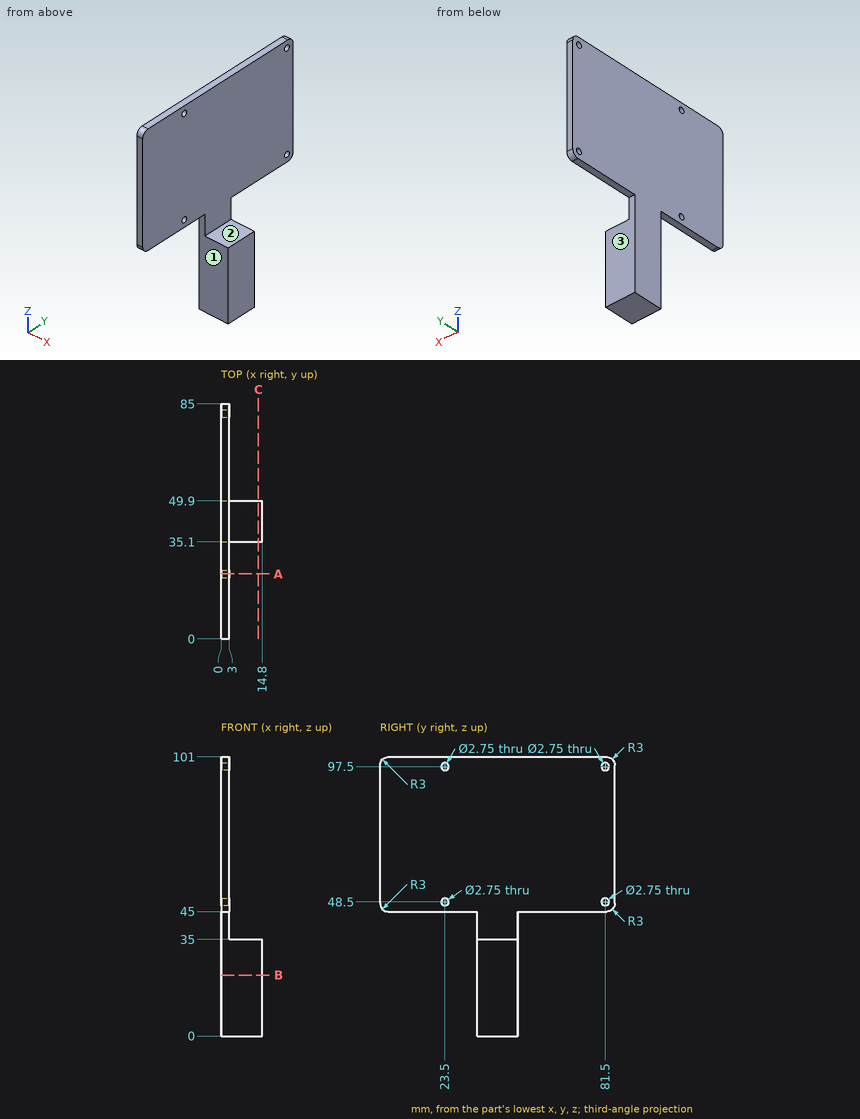
Answer from the drawing. Dimensions are ordinates in mm from the lowest x, y and z of the part. A direction names the side the tool comes from. Round coordinates to 2 decimals unless told otherwise and drop trailing zeros. Order: outer loops, then holes, each group sorted by start corner. A loop starts at its lowest first (then second) coordinate and runs counter-clockwise, first axis right, second up. Notation, with made-up numbers: (7.5, 74) - (57.5, 74) arc R15 cw to (57.5, 96) - close; hole circle Ø8 at (81.25, 32.25). An arc over 180 degrees is marked (long way). Put each result on its own line as item: value. Start each with the question number.
(1) Find section B-B (z = 22). Give the vertices of the cut face in (x, y).
(2) Given P1, Ø4, axis at x = 8.5, y = 41, coming from the +Z side; P2, Ø4, axis at y = 20, z = 77, coming from the +X side; P3, Ø3.5, axis at x = 1, y = 14.5, coming from the -Z side, each flat-ended and moving along its own axis, determine where each tip first touches the part or whether it passes through.
(3) Find section C-C (x = 13.5). Give the vertices of the cut face in (y, z), plus the area to 3 significant figures.
(4) For the marked faces 1, 2 and 3, determine the directions among +Z, -Z, +X, -X, +Y, -Y from which every point of the face is accessible in a straight line to the end or side of a thin tool.
(5) Find section A-A (y = 23.5). Give the vertices of the cut face in (x, z) (3 decimals).
(6) Straight lines are drawn through the part: probe 1 along Y at (x, z) = (2.25, 97.5) (3 decimals); probe 2 along Z at (x, y) = (1.6, 81.5) (3 decimals); probe 3 along X at (y, z) = (57, 81). For each, find the intervals that lie inside material, in ascending order. Write a range as from..to.
Reply:
1. outline: (0, 35.1) - (14.8, 35.1) - (14.8, 49.9) - (0, 49.9) - close
2. P1: z = 35
2. P2: x = 3
2. P3: z = 45
3. outline: (35.1, 0) - (49.9, 0) - (49.9, 35) - (35.1, 35) - close
3. area: 518 mm^2
4. face 1: -Z, +X, -X, -Y
4. face 2: +Z, +X, +Y, -Y
4. face 3: -Z, +X, -X, +Y
5. outline: (0, 45) - (3, 45) - (3, 47.125) - (0, 47.125) - close; (0, 49.875) - (3, 49.875) - (3, 96.125) - (0, 96.125) - close; (0, 98.875) - (3, 98.875) - (3, 101) - (0, 101) - close
6. probe 1: 0..22.125, 24.875..80.125, 82.875..85
6. probe 2: 45..47.125, 49.875..96.125, 98.875..101
6. probe 3: 0..3
